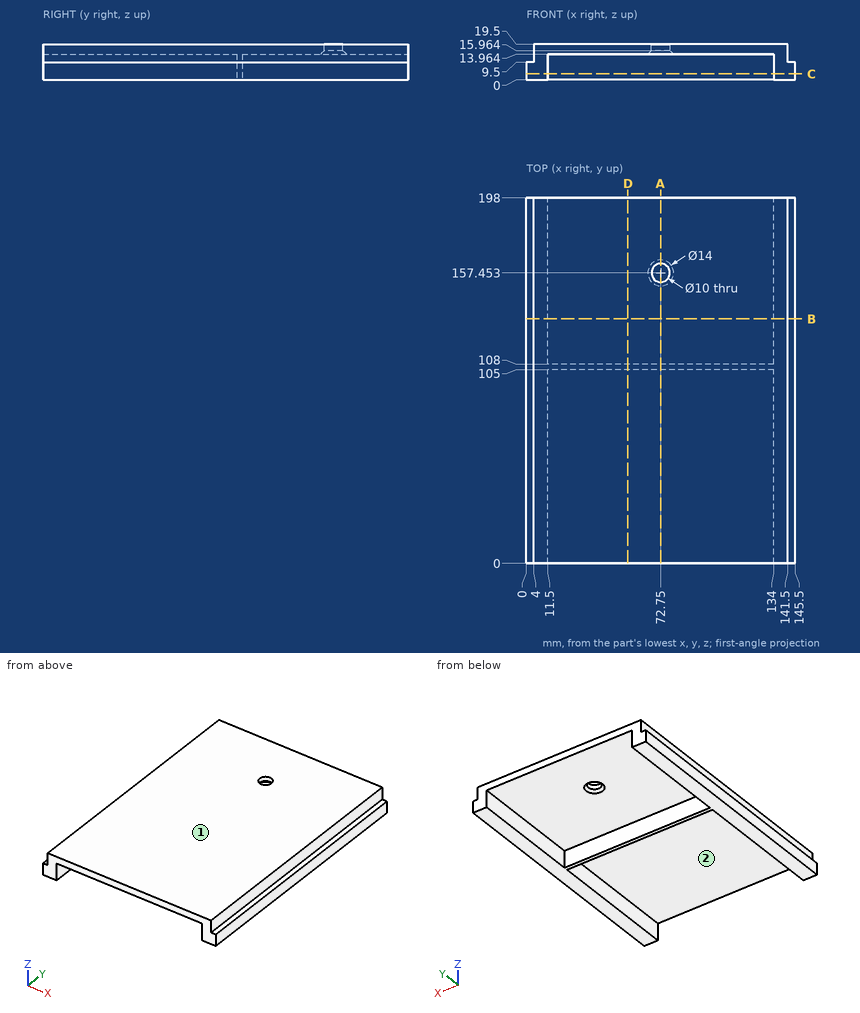
Job drawing, mm, ordinate dimensions from the low corner. One solid piece. Give positions to 0.01 mm unless a question says otherwise; leave off trailing zeros. Loops run counter-clockwise (first coordinate to the right, second up) from the corner with the lowest first, then second, coordinate; pieces in that order, holes last. Notation, with made-up numbers: (-30, 26) -> (-6, 26) arc R32 ccw to (-6, 57) -> close; hole circle Ø4 at (85.5, 47). An arc over 180 degrees is marked (long way). Write each question's results on one line, items separated by ' | '. Start each with the question number.
Q1. Pin check, flat tips, straight feed: P1, Ø1.2, axis at x = 143, y = 136.5, coming from the +Z side; P2, Ø3, axis at x = 114.5, z = 13.5, coming from the -Y side; P3, Ø4, axis at x = 90.5, z = 2, coming from the +Y side; P4, Ø13, axis at x = 72.75, y = 157.45, coming from the -Z side. Stop position of each tip, or through.
Q2. Band-saw the part on A-A on x = 72.75. List the corners of the cut face in (y, z), plus the area to 3 significant figures.
Q3. Wall check: L1, parallel to X at y = 86.5, z = 10.75; L2, parallel to Y at x = 72.75, z = 16.9; L3, parallel to X at y = 174, z = 8. Give the ranges that are in metal, low to high.
Q4. Band-saw the part on B-B on y = 132.5. List the corners of the cut face in (x, z), plus the area to 3 significant figures.
Q5. Band-saw the part on D-D on x = 55. List the corners of the cut face in (y, z), plus the area to 3 significant figures.
Q6. Band-saw the part on C-C on z = 3.25. List the corners of the cut face in (x, y).
Q7. Pull direction X, two halves, no side cores. Call the marked faces 1 and 2: +X half, -X half, draft (parallel to the pull), parting line (faces both ways), or undercut.
Results are:
1) P1: stops at z = 9.5 | P2: stops at y = 0 | P3: stops at y = 108 | P4: stops at z = 14.46
2) outline: (0, 13.96) -> (105, 13.96) -> (105, 0) -> (108, 0) -> (108, 13.96) -> (150.45, 13.96) -> (152.45, 15.96) -> (152.45, 19.5) -> (0, 19.5) -> close; (162.45, 15.96) -> (164.45, 13.96) -> (198, 13.96) -> (198, 19.5) -> (162.45, 19.5) -> close | area: 1,080 mm²
3) L1: x = 4 to 11.5, 134 to 141.5 | L2: y = 0 to 152.45, 162.45 to 198 | L3: x = 0 to 11.5, 134 to 145.5
4) outline: (0, 0) -> (11.5, 0) -> (11.5, 13.96) -> (134, 13.96) -> (134, 0) -> (145.5, 0) -> (145.5, 9.5) -> (141.5, 9.5) -> (141.5, 19.5) -> (4, 19.5) -> (4, 9.5) -> (0, 9.5) -> close | area: 1,050 mm²
5) outline: (0, 13.96) -> (105, 13.96) -> (105, 0) -> (108, 0) -> (108, 13.96) -> (198, 13.96) -> (198, 19.5) -> (0, 19.5) -> close | area: 1,140 mm²
6) outline: (0, 0) -> (11.5, 0) -> (11.5, 105) -> (134, 105) -> (134, 0) -> (145.5, 0) -> (145.5, 198) -> (134, 198) -> (134, 108) -> (11.5, 108) -> (11.5, 198) -> (0, 198) -> close
7) face 1: draft | face 2: undercut
